```python
from build123d import *

# Parameters (mm, degrees)
F1_DEPTH = 10


with BuildPart() as f1:
    # F0 (on Top) → F1 (new body)
    with BuildSketch(Plane.XY):
        Polygon((-44.130353, 14.681706), (-44.130353, 1.213891), (-41.730353, 1.213891), (-41.730353, 18.681706), (-44.130353, 18.681706), align=None)
        with BuildLine():
            Line((-45.730353, 14.681706), (-44.130353, 14.681706))
            Line((-44.130353, 14.681706), (-44.130353, 18.681706))
            ThreePointArc((-44.130353, 18.681706), (-45.261724, 18.213077), (-45.730353, 17.081706))
            Line((-45.730353, 17.081706), (-45.730353, 14.681706))
        make_face()
    extrude(amount=-F1_DEPTH)


solid = f1.part
```
Work out the finished part from the listing and answer in its coordinate system (mm). A direction names the side the tool comes from. Give positions to 0.01 mm unless a question says otherwise; leave off trailing zeros. Order: outer loops, then holes, each group sorted by start corner. A loop starts at its lowest first (then second) coordinate and runs counter-clockwise, first axis right, second up.
1. Each of these flat-tipped pins is pushed along its axis until it touches: P1, Ø1.5, axis at x = -45, y = 5.5, coming from the +Z side; P2, Ø5, axis at y = 10, z = -5, coming from the -X side. Where does it stop, or does it pass through?
Result sheet:
P1: passes through
P2: stops at x = -44.13
2. For faces 1 (the flat face through (-44.13, 8, -5)), 2 (the flat face through (-43, 12, 0)), determine the directions among +Z, -Z, +X, -X, +Y, -Y from which every point of the face is accessible in a straight line to the end or side of a thin tool.
Result sheet:
face 1: +Z, -Z, -X, -Y
face 2: +Z, +X, -X, +Y, -Y
3. Section B-B, the plane y = 9.5 is taken. Determine the outline of the cut face in (x, z).
Result sheet:
outline: (-44.13, -10) - (-41.73, -10) - (-41.73, 0) - (-44.13, 0) - close
4. Section C-C, the plane x = -45.2 is taken. Determine the outline of the cut face in (y, z), and give its area (3 significant figures).
Result sheet:
outline: (14.68, -10) - (18.27, -10) - (18.27, 0) - (14.68, 0) - close
area: 35.9 mm2
5. Section A-A, the plane z = -6.5 is taken. Determine the outline of the cut face in (x, y), and give its area (3 significant figures).
Result sheet:
outline: (-45.73, 14.68) - (-44.13, 14.68) - (-44.13, 1.21) - (-41.73, 1.21) - (-41.73, 18.68) - (-44.13, 18.68) arc R1.6 ccw to (-45.73, 17.08) - close
area: 47.8 mm2
6. Straight lines are drawn through the part: L1, parallel to X at y = 5.75, z = -9.5; L2, parallel to Y at x = -45.45, z = -9; L3, parallel to Y at x = -44.8, z = -4.75. For each, find the intervals that lie inside material, in ascending order.
Result sheet:
L1: x = -44.13 to -41.73
L2: y = 14.68 to 17.99
L3: y = 14.68 to 18.53
